Check sheet for the drawn part. Datum: minimum x, y, z corner. Units: mm. A direction names the side the tool comes from. Give positions to 0.01 mm unless a question says otherwise; leave off trailing zeros. Write each loop counter-clockwise with the first axis right and the second up, starting at its lowest first coordinate (ties: lowest second). Pieces come first, ordered by that corner, then holes.
(1) Depth check by flat-ended pin: P1, Ø5, axis at y = 9, z = 19, coming from the +X side (1 decimal); P2, Ø6.5, axis at y = 4.5, z = 76.5, coming from the -X side; P3, Ø2.5, axis at x = 2.5, y = 4.5, coming from the -Z side; P4, Ø7.5, axis at x = 36.51, z = 79.38, coming from the -Y side. Enter the tip coordinate at first touch or a pass-through.
(2) Tool access check on the marked faces 4, 5, 6, 7 and 8. Record the directions out of +Z, -Z, +X, -X, +Y, -Y that give a thin tool (end or side, any length) a straight path to the whole face; none if there is none.
(3) Cross-section at D-D (y = 10.5). Count the separate pieces of the cut face and the enclosed holes in it, and give its area (3 significant figures).
(4) Cross-section at C-C (x = 65). Record the boundary of the cut face in (y, z) (1 decimal).
(5) Mould release check, pull along X, two halves, no side actions. Record for the marked faces 1, 2 and 3: +X half, -X half, draft (parallel to the pull), parting line (faces both ways), or undercut.
(6) Thickness scan on line 1 along X through (y, z) = (4, 69.5) (1 decimal); line 2 along X through (y, z) = (10.5, 54) (1 decimal); line 3 along X through (y, z) = (2, 28) (1 decimal). Record the ranges inside material, lowest first.
(7) Cross-section at A-A (z = 11). Record the boundary of the cut face in (x, y).
(8) Cross-section at B-B (z = 63). Record the boundary of the cut face in (x, y) (1 decimal).
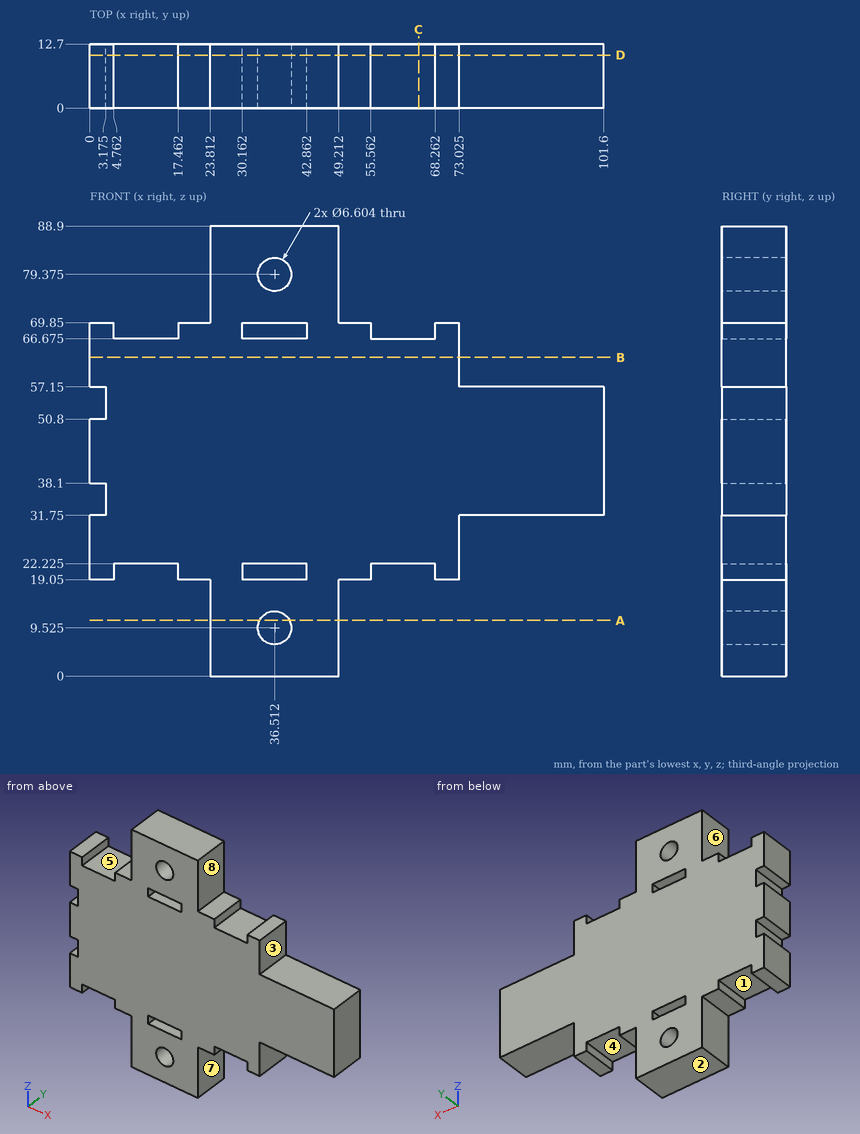
Reply:
1. P1: stops at x = 73
1. P2: stops at x = 23.81
1. P3: stops at z = 19.05
1. P4: stops at y = 0
2. face 4: -Z, +Y, -Y
2. face 5: +Z, +Y, -Y
2. face 6: +Z, -X, +Y, -Y
2. face 7: -Z, +X, +Y, -Y
2. face 8: +Z, +X, +Y, -Y
3. separate pieces: 1
3. enclosed holes: 4
3. area: 5,050 mm2
4. outline: (0, 22.2) - (12.7, 22.2) - (12.7, 66.7) - (0, 66.7) - close
5. face 1: undercut
5. face 2: draft
5. face 3: +X half
6. line 1: x = 0 to 4.8, 17.5 to 30.2, 42.9 to 55.6, 68.3 to 73
6. line 2: x = 3.2 to 101.6
6. line 3: x = 0 to 73
7. outline: (23.81, 0) - (33.56, 0) - (33.56, 12.7) - (23.81, 12.7) - close; (39.47, 0) - (49.21, 0) - (49.21, 12.7) - (39.47, 12.7) - close
8. outline: (0, 0) - (73, 0) - (73, 12.7) - (0, 12.7) - close
